```python
from build123d import *

# Parameters (mm, degrees)
SKETCH1_R           = 26.5
BOSS_EXTRUDE1_DEPTH = 2
CUT_EXTRUDE1_START  = -2
CUT_EXTRUDE1_DEPTH  = 2
CIRPATTERN2_COUNT   = 25
CUT_EXTRUDE2_DEPTH  = 2


with BuildPart() as part:
    # Sketch1 → Boss-Extrude1 (new body)
    with BuildSketch(Plane(origin=(0, 0, 0), x_dir=(1, 0, 0), z_dir=(0, 1, 0))):
        with Locations(Location((0, 0, 0), (0, 0, 270))):
            Circle(SKETCH1_R)
    extrude(amount=BOSS_EXTRUDE1_DEPTH)

    # Sketch2 → Cut-Extrude1 (cut)
    with BuildSketch(Plane(origin=(0, 2, 0), x_dir=(1, 0, 0), z_dir=(0, 1, 0)).offset(CUT_EXTRUDE1_START)):
        with BuildLine():
            ThreePointArc((20.67056927, 16.582447529), (18.581221902, 18.894131169), (16.234972011, 20.944586026))
            add(Edge.make_bspline(
                [(16.234972011, 20.944586026), (12.135241932, 12.33960038), (20.67056927, 16.582447529)],
                knots=[0, 0, 0, 1, 1, 1], degree=2, weights=[1, 0.580612476, 1]))
        make_face()
    cut_extrude1 = extrude(amount=CUT_EXTRUDE1_DEPTH, mode=Mode.SUBTRACT)

    # CirPattern2: Cut-Extrude1 ×25 about axis
    cirpattern2_axis = Axis((0, 2, 0), (0, -1, 0))
    for i in range(1, CIRPATTERN2_COUNT):
        add(cut_extrude1.rotate(cirpattern2_axis, i * 360 / CIRPATTERN2_COUNT), mode=Mode.SUBTRACT)

    # Sketch4 → Cut-Extrude2 (cut)
    with BuildSketch(Plane(origin=(0, 2, 0), x_dir=(1, 0, 0), z_dir=(0, 1, 0))):
        with BuildLine():
            Line((2.645751311, -3), (-2.645751311, -3))
            ThreePointArc((-2.645751311, -3), (0, 4), (2.645751311, -3))
        make_face()
    extrude(amount=-CUT_EXTRUDE2_DEPTH, mode=Mode.SUBTRACT)


solid = part.part
```
Model file for the job. Use its own axes, mm. A direction names the side the tool comes from. Coordinates: 2 decimals unless noted, no trailing zeros. Answer as a JSON object with one key per item and string values. Group by question number.
1) Drill centre lines: L1, parallel to Z at x = -23.5, y = 1.4; L2, parallel to X at y = 1.2, z = -7; L3, parallel to X at y = 1.45, z = 0. Where is each one in solid material? Low to high.
2) Pull direction Z, two halves, no side cores. Call faces 3 (the face through (0, 1, -4)), 4 (the face through (0, 2, 6)): +Z half, -Z half, draft (parallel to the pull), parting line (faces both ways), or undercut.
3) Flat gauge pins, fed straight in: pin 1 (0.6 mm diameter, centred on x = 1, y = 0.5, fed in from -Z); pin 2 (1 mm diameter, centred on x = 16.5, y = 1.5, fed in from -Z). Where does each tip first touch, or does it go through?
4) Which spindle directions (+Z, -Z, +X, -X, +Y, -Y) get a long thin tool onto all of the face, cutting with end or side? Do faces 1 (the face through (0, 0, 6)), 2 (the face through (0, 1, 3)). Say none if no direction does.
Check values:
{
 "1": {"L1": "z = -11.99 to -11.39, -6.1 to -3.62, -0.72 to 2.47, 5.94 to 7.84", "L2": "x = -22.07 to 21.97", "L3": "x = -24.39 to -4, 4 to 23.26"},
 "2": {"face 3": "undercut", "face 4": "draft"},
 "3": {"pin 1": "stops at z = -23.14", "pin 2": "stops at z = -21.12"},
 "4": {"face 1": "+Z, -Z, +X, -X, -Y", "face 2": "+Y, -Y"}
}
